from build123d import *

# Parameters (mm, degrees)
BOSS_EXTRUDE1_DEPTH = 30
SKETCH2_W           = 60
SKETCH2_H           = 41.5
CUT_EXTRUDE1_DEPTH  = 27
SKETCH5_W           = 60
SKETCH5_H           = 3
BOSS_EXTRUDE2_DEPTH = 15
FILLET2_R           = 1
FILLET3_R           = 3
FILLET4_R           = 3
CUT_EXTRUDE2_START  = 14
CUT_EXTRUDE2_DEPTH  = 5
CUT_EXTRUDE3_START  = -30
SKETCH7_R           = 1.25
CUT_EXTRUDE3_DEPTH  = 25
SKETCH8_R           = 2.5
CUT_EXTRUDE4_DEPTH  = 4
SKETCH9_R           = 6.5
CUT_EXTRUDE5_DEPTH  = 1.75
SKETCH10_R          = 2
CUT_EXTRUDE6_DEPTH  = 31
SKETCH11_R          = 3.5
CUT_EXTRUDE7_DEPTH  = 10


with BuildPart() as part:
    # Sketch1 → Boss-Extrude1 (new body)
    with BuildSketch(Plane.XY):
        with BuildLine():
            Line((-18, 25), (18, 25))
            ThreePointArc((18, 25), (43, 0), (18, -25))
            Line((18, -25), (-18, -25))
            ThreePointArc((-18, -25), (-43, 0), (-18, 25))
        make_face()
    extrude(amount=BOSS_EXTRUDE1_DEPTH)

    # Sketch2 → Cut-Extrude1 (cut)
    with BuildSketch(Plane.XY.offset(30)):
        Rectangle(SKETCH2_W, SKETCH2_H)
    extrude(amount=-CUT_EXTRUDE1_DEPTH, mode=Mode.SUBTRACT)

    # Sketch5 → Boss-Extrude2 (add)
    with BuildSketch(Plane.XY.offset(3)):
        with Locations((0, 19.25)):
            Rectangle(SKETCH5_W, SKETCH5_H)
        with Locations((0, -19.25)):
            Rectangle(SKETCH5_W, SKETCH5_H)
    extrude(amount=BOSS_EXTRUDE2_DEPTH)

    # Fillet2
    fillet2_edges = [part.edges().sort_by_distance(p)[0] for p in [
        (-30, 20.75, 24),
        (30, 20.75, 24),
        (30, -20.75, 24),
        (-30, -20.75, 24),
    ]]
    fillet(fillet2_edges, radius=FILLET2_R)

    # Fillet3
    fillet3_edges = [part.edges().sort_by_distance(p)[0] for p in [
        (-30, 0, 3),
        (0, 17.75, 3),
        (30, 0, 3),
        (0, -17.75, 3),
    ]]
    fillet(fillet3_edges, radius=FILLET3_R)

    # Fillet4
    fillet4_edges = [part.edges().sort_by_distance(p)[0] for p in [
        (0, 25, 0),
        (43, 0, 0),
        (0, -25, 0),
        (-43, 0, 0),
    ]]
    fillet(fillet4_edges, radius=FILLET4_R)

    # Sketch6 → Cut-Extrude2 (cut)
    with BuildSketch(Plane.XY.offset(CUT_EXTRUDE2_START)):
        with BuildLine():
            Line((-44.296401613, 12), (-33, 12))
            ThreePointArc((-33, 12), (-30.878679656, 12.878679656), (-30, 15))
            Line((-30, 15), (-30, 24.104241325))
            Line((-30, 24.104241325), (-44.296401613, 12))
        make_face()
        with BuildLine():
            Line((30, 24.104241325), (44.296401613, 12))
            Line((44.296401613, 12), (33, 12))
            ThreePointArc((33, 12), (30.878679656, 12.878679656), (30, 15))
            Line((30, 15), (30, 24.104241325))
        make_face()
    extrude(amount=CUT_EXTRUDE2_DEPTH, mode=Mode.SUBTRACT)

    # Sketch7 → Cut-Extrude3 (cut)
    with BuildSketch(Plane(origin=(0, 0, 0), x_dir=(-1, 0, 0), z_dir=(0, 0, -1)).offset(CUT_EXTRUDE3_START)):
        with Locations((-33, 15)):
            Circle(SKETCH7_R)
    cut_extrude3 = extrude(amount=CUT_EXTRUDE3_DEPTH, mode=Mode.SUBTRACT)

    # Sketch8 → Cut-Extrude4 (cut)
    with BuildSketch(Plane.XY.offset(30)):
        with Locations((33, 15)):
            Circle(SKETCH8_R)
    cut_extrude4 = extrude(amount=-CUT_EXTRUDE4_DEPTH, mode=Mode.SUBTRACT)

    # Mirror1: Cut-Extrude3, Cut-Extrude4 across plane
    add(cut_extrude3.mirror(Plane(origin=(0, 0, 0), x_dir=(0, 0, 1), z_dir=(1, 0, 0))), mode=Mode.SUBTRACT)
    add(cut_extrude4.mirror(Plane(origin=(0, 0, 0), x_dir=(0, 0, 1), z_dir=(1, 0, 0))), mode=Mode.SUBTRACT)

    # Sketch9 → Cut-Extrude5 (cut)
    with BuildSketch(Plane.XY.offset(3)):
        with Locations((-15, 0)):
            Circle(SKETCH9_R)
        with Locations((15, 0)):
            Circle(SKETCH9_R)
    extrude(amount=-CUT_EXTRUDE5_DEPTH, mode=Mode.SUBTRACT)

    # Sketch10 → Cut-Extrude6 (cut, through all)
    with BuildSketch(Plane(origin=(0, 0, 0), x_dir=(-1, 0, 0), z_dir=(0, 0, -1))):
        with Locations((-34, 8)):
            Circle(SKETCH10_R)
        with Locations((34, 8)):
            Circle(SKETCH10_R)
    extrude(amount=-CUT_EXTRUDE6_DEPTH, mode=Mode.SUBTRACT)

    # Sketch11 → Cut-Extrude7 (cut)
    with BuildSketch(Plane(origin=(0, 0, 0), x_dir=(-1, 0, 0), z_dir=(0, 0, -1))):
        with Locations((-34, 8)):
            Circle(SKETCH11_R)
        with Locations((34, 8)):
            Circle(SKETCH11_R)
    extrude(amount=-CUT_EXTRUDE7_DEPTH, mode=Mode.SUBTRACT)


solid = part.part
Input: part model. Units: mm. Frame: model coordinates. A direction names the side the tool comes from. Coordinates: 2 decimals unless noted, no trailing zeros. Loops run counter-clockwise (first coordinate to the right, second up) from the corner with the lowest first, then second, coordinate; pieces in that order, holes last. Notation, with made-up numbers: (32.25, 49.5) -> (61.25, 49.5) arc R13 cw to (61.25, 65.5) -> close; hole circle Ø6 at (75, 79). An arc over 180 degrees is marked (long way). Write item = value, one per line. Start each with the question number.
Item 1: Material intervals for line 1 (Y direction, x = 2.5, z = 27.25); line 2 (X direction, y = 7, z = 5.25); line 3 (Y direction, x = 33, z = 29.15), sorted ascending.
Item 2: Cut plane A-A, the plane z = 16.25. Return loops of the section in (x, y).
Item 3: First-contact query: P1, Ø8, axis at y = -15, z = 4.5, coming from the +X side; P2, Ø8, axis at y = -9.5, z = 4.5, coming from the -X side; P3, Ø5, axis at x = -34, z = 9.5, coming from the +Y side; P4, Ø2, axis at x = 33.5, y = 8.5, coming from the -Z side. Flat tips, straight axial feed; report the tip coordinate or a pass-through.
Item 4: Reachability of faces 1 (the face through (-30, 20, 16)), 2 (the face through (30.9, 12.86, 16.46)), 3 (the face through (-33.241, 4.583, 4.93)), 4 (the face through (0, 0, 3)) from +Z, -Z, +X, -X, +Y, -Y: full face, straight path, thin tool, end or side. Return the list, or none.
Item 5: Cut plane D-D, the plane x = -15. Return loops of the section in (y, z), plus the area to 3 significant figures.
Item 6: Cut plane C-C, the plane y = 0. Return loops of the section in (x, z).
Item 7: Cut plane B-B, the plane z = 21. Return loops of the section in (x, y).
Item 8: Mould query, pull axis Y, two halves, no side actions, for faces 5 (the face through (0, -25, 16)), 6 (the face through (-30.9, 12.86, 16.46)), 7 (the face through (-15, 0, 1.25)). Classes: pulls with the +Y half, pulls with the -Y half, needs draft (parallel to the pull), parting line crosses it, or undercut.
Ans:
q1.line_1 = -25 to -20.75, 20.75 to 25
q1.line_2 = -42 to -37.35, -30.65 to -29.9, 29.9 to 30.65, 37.35 to 42
q1.line_3 = -20 to 6.27, 9.73 to 12.5, 17.5 to 20
q2.outline = (-39.93, 12) arc R25 ccw to (-18, -25) -> (18, -25) arc R25 ccw to (39.93, 12) -> (33, 12) arc R3 cw to (30, 15) -> (30, -17.75) -> (-30, -17.75) -> (-30, 15) arc R3 cw to (-33, 12) -> close; (-30, 17.75) -> (30, 17.75) -> (30, 21.93) arc R25 ccw to (18, 25) -> (-18, 25) arc R25 ccw to (-30, 21.93) -> close; hole circle Ø4 at (-34, 8); hole circle Ø4 at (34, 8)
q3.P1 = 40.45
q3.P2 = -42.39
q3.P3 = 21.04
q3.P4 = through
q4.face_1 = -X, +Y
q4.face_2 = +X, +Y
q4.face_3 = -Z
q4.face_4 = +Z
q5.outline = (-25, 3) arc R3 ccw to (-22, 0) -> (22, 0) arc R3 ccw to (25, 3) -> (25, 30) -> (20.75, 30) -> (20.75, 18) -> (17.75, 18) -> (17.75, 6) arc R3 cw to (14.75, 3) -> (6.5, 3) -> (6.5, 1.25) -> (-6.5, 1.25) -> (-6.5, 3) -> (-14.75, 3) arc R3 cw to (-17.75, 6) -> (-17.75, 18) -> (-20.75, 18) -> (-20.75, 30) -> (-25, 30) -> close
q5.area = 447 mm²
q6.outline = (-43, 3) arc R3 ccw to (-40, 0) -> (40, 0) arc R3 ccw to (43, 3) -> (43, 30) -> (30, 30) -> (30, 6) arc R3 cw to (27, 3) -> (21.5, 3) -> (21.5, 1.25) -> (8.5, 1.25) -> (8.5, 3) -> (-8.5, 3) -> (-8.5, 1.25) -> (-21.5, 1.25) -> (-21.5, 3) -> (-27, 3) arc R3 cw to (-30, 6) -> (-30, 30) -> (-43, 30) -> close
q7.outline = (-18, -25) -> (18, -25) arc R25 ccw to (18, 25) -> (-18, 25) arc R25 ccw to start; hole circle Ø4 at (-34, 8); hole circle Ø2.5 at (-33, 15); hole (-30, -19.75) arc R1 ccw to (-29, -20.75) -> (29, -20.75) arc R1 ccw to (30, -19.75) -> (30, 19.75) arc R1 ccw to (29, 20.75) -> (-29, 20.75) arc R1 ccw to (-30, 19.75) -> close; hole circle Ø2.5 at (33, 15); hole circle Ø4 at (34, 8)
q8.face_5 = pulls with the -Y half
q8.face_6 = pulls with the +Y half
q8.face_7 = undercut
